Input: part model. Units: mm. Frame: model coordinates. A direction names the side the tool comes from. Round coordinates to 2 decimals unless told otherwise and drop trailing zeros. Loops run counter-clockwise (first coordinate to the right, second up) from the corner with the lowest first, then second, coordinate; pieces in that order, holes last. Notation, with made-up numbers: (51.25, -4) - (92.25, -4) arc R33 ccw to (92.25, 25) - close; hole circle Ø11 at (67.5, 24.25). An arc over 180 degrees is marked (long way). Write each question's results on one line, items separated by ' | '.
Autodesk Inventor part; units mm, degrees
ref_plane "YZ Plane" through (0, 0, 0) normal (1, 0, 0) x (0, 1, 0)
ref_plane "XZ Plane" through (0, 0, 0) normal (0, 1, 0) x (-1, 0, 0)
ref_plane "XY Plane" through (0, 0, 0) normal (0, 0, 1) x (1, 0, 0)
sketch "Sketch1" plane through (0, 0, 0) normal (0, 0, 1) x (1, 0, 0)
  line L0 (98, 0) -> (98, -90)
  line L1 (98, -90) -> (-90, -90)
  line L2 (-90, -90) -> (-90, 0)
  line L3 (126, 4) -> (126, 0)
  line L4 (126, 0) -> (-118, 0)
  line L5 (-118, 0) -> (-118, 4)
  line L6 (-86, 4) -> (94, 4)
  line L7 (94, 4) -> (94, -86)
  line L8 (94, -86) -> (-86, -86)
  line L9 (-86, -86) -> (-86, 4)
  line L10 (-90, 0) -> (-86, 0)
  line L11 (94, 0) -> (98, 0)
  line L12 (-118, 4) -> (-86, 4)
  line L13 (94, 4) -> (126, 4)
  point P0 (0, 0)
  point P1 (6, -4)
  point P2 (126, 2)
  point P3 (98, 0)
  dimension "d0" = 188
  dimension "d1" = 90
  dimension "d3" = 90
  dimension "d4" = 244
  dimension "d5" = 120
  dimension "d8" = 90
  dimension "d9" = 180
  dimension "d10" = 4
  dimension "d13" = 0
  dimension "d14" = 4
  dimension "d90" = 32
extrude "Extrusion1" add sketch "Sketch1" along normal blind 250 contours L4 L7 L13 L3 | L0 L1 L2 L4 L9 L8 L7 | L4 L5 L12 L9
fillet "Fillet1" radius 2 4 edges at (-86, -86, 125) (-86, 4, 125) (94, 4, 125) (98, -90, 125)
fillet "Fillet2" radius 2 2 edges at (-90, -90, 125) (94, -86, 125)
sketch "Sketch3" plane through (-84, -86, 250) normal (0, 1, 0) x (1, 0, 0)
  line L0 (-2, 0) -> (-2, 250)
  line L1 (176, 0) -> (0, 0)
  point P0 (84, 250)
  point P1 (114.75, 74.7)
  point P2 (61.25, 74.7)
  dimension "d28" = 53.5
  dimension "d29" = 63.25
  dimension "d30" = 0
  dimension "d31" = 74.7
hole "Hole2" at (30.75, -86, 175.3) at (-22.75, -86, 175.3) direction (0, -1, 0) diameter 3.4587 end through all
sketch "Sketch4" plane through (-84, -86, 250) normal (0, 1, 0) x (1, 0, 0)
  circle A0 centre (61.25, 74.7) radius 1.7294
  circle A1 centre (114.75, 74.7) radius 1.7294
  point P0 (84, 250)
  point P1 (114.75, 142.7)
  point P2 (61.25, 142.7)
  dimension "d39" = 53.5
  dimension "d40" = 68
  dimension "d41" = 68
  dimension "d49" = 0
hole "Hole3" at (30.75, -86, 107.3) at (-22.75, -86, 107.3) direction (0, -1, 0) diameter 3.4587 end through all
sketch "Sketch5" plane through (-84, -86, 250) normal (0, 1, 0) x (1, 0, 0)
  circle A0 centre (61.25, 74.7) radius 1.7294
  circle A1 centre (114.75, 74.7) radius 1.7294
  circle A2 centre (61.25, 142.7) radius 1.7294
  point P0 (84, 250)
  point P1 (71, 91.2)
  point P2 (71, 126.2)
  point P3 (106, 126.2)
  point P4 (106, 91.2)
  dimension "d50" = 35
  dimension "d51" = 35
  dimension "d52" = 35
  dimension "d53" = 16.5
  dimension "d54" = 16.5
  dimension "d55" = 9.75
hole "Hole4" at (-13, -86, 158.8) at (-13, -86, 123.8) at (22, -86, 123.8) at (22, -86, 158.8) direction (0, -1, 0) diameter 3.4587 end through all
sketch "Sketch6" plane through (-84, -86, 250) normal (0, 1, 0) x (1, 0, 0)
  circle A0 centre (71, 126.2) radius 1.7294
  point P0 (84, 250)
  point P1 (88.5, 108.7)
  dimension "d63" = 17.5
  dimension "d64" = 17.5
hole "Hole5" at (4.5, -86, 141.3) direction (0, -1, 0) diameter 3 end through all
sketch "Sketch7" plane through (126, 4, 250) normal (0, 1, 0) x (1, 0, 0)
  line L0 (-244, 250) -> (-244, 0)
  line L1 (-214, 0) -> (-244, 0)
  line L2 (-214, 250) -> (-244, 250)
  line L3 (0, 250) -> (0, 0)
  line L4 (0, 250) -> (-30, 250)
  line L5 (-28, 0) -> (0, 0)
  point P0 (-126, 250)
  point P1 (-228, 20)
  point P2 (-228, 60)
  point P3 (-228, 230.025)
  point P4 (-228, 190.025)
  point P5 (-228, 150.025)
  point P6 (-16, 230)
  point P7 (-16, 190)
  point P8 (-16, 150)
  point P9 (-16, 60)
  point P10 (-16, 20)
  point P11 (-229, 250)
  point P12 (-15, 250)
  dimension "d72" = 16
  dimension "d73" = 16
  dimension "d74" = 16
  dimension "d75" = 16
  dimension "d76" = 16
  dimension "d77" = 20
  dimension "d78" = 40
  dimension "d79" = 20
  dimension "d80" = 40
  dimension "d81" = 40
  dimension "d82" = 16
  dimension "d83" = 16
  dimension "d84" = 16
  dimension "d85" = 16
  dimension "d86" = 16
  dimension "d87" = 20
  dimension "d88" = 40
  dimension "d89" = 40
  dimension "d98" = 20
  dimension "d99" = 40
hole "Hole6" at (-102, 4, 230) at (-102, 4, 190) at (-102, 4, 19.975) at (-102, 4, 59.975) at (-102, 4, 99.975) at (110, 4, 20) at (110, 4, 60) at (110, 4, 100) at (110, 4, 190) at (110, 4, 230) direction (0, -1, 0) diameter 4.917 end through all
equation "\"BendRadius\" = Thickness"
equation "\"BendReliefWidth\" = Thickness"
equation "\"BendReliefDepth\" = 0.5 * Thickness"
equation "\"CornerReliefSize\" = 4 * Thickness"
equation "\"MinimumRemnant\" = 2 * Thickness"
equation "\"TransitionRadius\" = BendRadius"
equation "\"JacobiRadiusSize\" = BendRadius"
equation "\"GapSize\" = Thickness"
properties part number "Lower joint housing"
1. Mould query, pull axis X, two halves, no side actions, for faces 6 (the flat face through (-103, 4, 123)), 7 (the flat face through (94, -40, 123)), 8 (the flat face through (98, -43, 123)). Classes: pulls with the +X half, pulls with the -X half, needs draft (parallel to the pull), parting line crosses it, or undercut.
Answer:
face 6: needs draft | face 7: undercut | face 8: pulls with the +X half
2. Section query A-A, the plane y = -22.5. Output: boundary loops of the cut face in (x, z).
Answer:
outline: (-90, 0) - (-86, 0) - (-86, 250) - (-90, 250) - close; (94, 0) - (98, 0) - (98, 250) - (94, 250) - close
3. Contact query for flat-ended pins moving along their axis: pin 1 (8 mm diameter, centred on x = -102, z = 19.975, fed in from -Y); pin 2 (2.5 mm diameter, centred on x = 4.5, z = 141.3, fed in from +Y); pin 3 (4 mm diameter, centred on x = 22, z = 158.8, fed in from +Y); pin 4 (8 mm diameter, centred on y = -60, z = 63, fed in from -X). Output: stop coordinate, or through.
Answer:
pin 1: y = 0 | pin 2: through | pin 3: y = -86 | pin 4: x = -90
4. Section query C-C, the plane x = 56. Output: boundary loops of the cut face in (y, z), plus the area to 3 significant figures.
Answer:
outline: (-90, 0) - (-86, 0) - (-86, 250) - (-90, 250) - close | area: 1,000 mm^2
5. Line query: line 1 (Z direction, x = -102, y = 1.1); line 2 (Z direction, x = 110, y = 2.15); line 3 (Z direction, x = 22, y = -86.95). Output: solid intervals per line, ascending. Write a range as [from, to].
Answer:
line 1: [0, 17.52], [22.43, 57.52], [62.43, 97.52], [102.43, 187.54], [192.46, 227.54], [232.46, 250] | line 2: [0, 17.54], [22.46, 57.54], [62.46, 97.54], [102.46, 187.54], [192.46, 227.54], [232.46, 250] | line 3: [0, 122.07], [125.53, 157.07], [160.53, 250]
6. Set-up query: faces 1 (the flat face through (-42, -88, 250)), 2 (the flat face through (-90, -45, 123)), 3 (the flat face through (112, 0, 123)), 4 (the flat face through (5, -90, 123)), 5 (the flat face through (5, -86, 123)). Return all of +Z, -Z, +X, -X, +Y, -Y with unobstructed straight access to the full face (end or side cutting, diameter ignored); none if empty.
Answer:
face 1: +Z, +X, -X, +Y, -Y | face 2: +Z, -Z, -X, -Y | face 3: +Z, -Z, +X, -Y | face 4: +Z, -Z, +X, -X, -Y | face 5: +Z, -Z, +Y
7. Section query B-B, the plane z = 221. Output: boundary loops of the cut face in (x, y).
Answer:
outline: (-118, 0) - (-90, 0) - (-90, -88) arc R2 ccw to (-88, -90) - (96, -90) arc R2 ccw to (98, -88) - (98, 0) - (126, 0) - (126, 4) - (96, 4) arc R2 ccw to (94, 2) - (94, -84) arc R2 cw to (92, -86) - (-84, -86) arc R2 cw to (-86, -84) - (-86, 2) arc R2 ccw to (-88, 4) - (-118, 4) - close
